from build123d import *

# Parameters (mm, degrees)
SKETCH1_R           = 5
BOSS_EXTRUDE1_DEPTH = 11
CUT_EXTRUDE1_DEPTH  = 8
BOSS_EXTRUDE2_DEPTH = 7


with BuildPart() as part:
    # Sketch1 → Boss-Extrude1 (new body)
    with BuildSketch(Plane.XY):
        with Locations((-12.317334514, -23.116112266)):
            Circle(SKETCH1_R)
    extrude(amount=BOSS_EXTRUDE1_DEPTH)

    # Sketch2 → Cut-Extrude1 (cut)
    with BuildSketch(Plane.XY.offset(11)):
        with BuildLine():
            Line((-14.317334514, -24.366112266), (-14.317334514, -21.866112266))
            ThreePointArc((-14.317334514, -21.866112266), (-12.317334514, -19.866112266), (-10.317334514, -21.866112266))
            Line((-10.317334514, -21.866112266), (-10.317334514, -24.366112266))
            ThreePointArc((-10.317334514, -24.366112266), (-12.317334514, -26.366112266), (-14.317334514, -24.366112266))
        make_face()
    extrude(amount=-CUT_EXTRUDE1_DEPTH, mode=Mode.SUBTRACT)

    # Sketch4 → Boss-Extrude2 (add)
    with BuildSketch(Plane(origin=(0, 0, 0), x_dir=(-1, 0, 0), z_dir=(0, 0, -1))):
        with BuildLine():
            Line((10.442334514, -24.116112266), (10.442334514, -22.116112266))
            ThreePointArc((10.442334514, -22.116112266), (12.317334514, -20.241112266), (14.192334514, -22.116112266))
            Line((14.192334514, -22.116112266), (14.192334514, -24.116112266))
            ThreePointArc((14.192334514, -24.116112266), (12.317334514, -25.991112266), (10.442334514, -24.116112266))
        make_face()
    extrude(amount=BOSS_EXTRUDE2_DEPTH)


solid = part.part
Here's how the part is built. I have some questions about the finished solid (model axes, mm). A direction names the side the tool comes from. Coordinates: 2 decimals unless noted, no trailing zeros. Write each loop counter-clockwise with the first axis right and the second up, starting at its lowest first coordinate (ties: lowest second). Pieces come first, ordered by that corner, then holes.
Item 1: I want a section at B-B on z = -4.75. Write out the boundary of the cut face in (x, y) (3 decimals), and give its area (3 significant figures).
Item 2: On a 3-axis mill with a long thin cutter (end or side, diameter ignored), from which of +Z, -Z, +X, -X, +Y, -Y can I reach the whole of each face in a straight line? I mean faces 1 (the flat face through (-12, -23, 3)), 2 (the flat face through (-14.192, -23, -3)), 3 (the cylindrical face through (-12.36, -25.99, -3.45)). Say none if no direction works.
Item 3: I want a section at A-A on x = -13.75. Write out the boundary of the cut face in (y, z).
Item 4: Will these pins go through, and if not, where does the flat tip stop? pin 1 (0.6 mm diameter, centred on y = -23.5, z = -2.5, fed in from +X); pin 2 (1.6 mm diameter, centred on y = -22.5, z = -4.5, fed in from -X); pin 3 (2 mm diameter, centred on x = -13, y = -23.5, fed in from +Z); pin 4 (1.2 mm diameter, centred on y = -22.5, z = 6.5, fed in from -X).
Item 5: If I drill on line 1 (Z direction, x = -11.75, y = -26.5); line 2 (Z direction, x = -13.25, y = -22.25); line 3 (Y direction, x = -13.25, z = 5.5), over which ranges is the centre line in solid material (lowest first)?
Item 6: I want a section at D-D on z = 9.5. Write out the boundary of the cut face in (x, y).
Item 7: I want a section at C-C on y = -25.5. Write out the boundary of the cut face in (x, z), and give its area (3 significant figures).
Item 8: If we mould it in two halves opening along Y, with no side actions, what happens to faces 4 (the cylindrical face through (-12.28, -20.24, -3.45)), 5 (the flat face through (-10.317, -23, 7)), 6 (the flat face through (-12, -23, -7))? For each: +Y half, -Y half, draft (parallel to the pull), parting line (faces both ways), or undercut.
Findings below:
1. outline: (-14.192, -24.116) arc R1.875 ccw to (-10.442, -24.116) - (-10.442, -22.116) arc R1.875 ccw to (-14.192, -22.116) - close
1. area: 18.5 mm2
2. face 1: +Z
2. face 2: -Z, -X, +Y, -Y
2. face 3: -Z, -Y
3. outline: (-27.91, 0) - (-25.33, 0) - (-25.33, -7) - (-20.91, -7) - (-20.91, 0) - (-18.33, 0) - (-18.33, 11) - (-20.47, 11) - (-20.47, 3) - (-25.76, 3) - (-25.76, 11) - (-27.91, 11) - close
4. pin 1: stops at x = -10.44
4. pin 2: stops at x = -14.19
4. pin 3: stops at z = 3
4. pin 4: stops at x = -17.32
5. line 1: z = 0 to 11
5. line 2: z = -7 to 3
5. line 3: y = -28.03 to -26.14, -20.1 to -18.2
6. outline: circle Ø10 at (-12.32, -23.12); hole (-14.32, -24.37) arc R2 ccw to (-10.32, -24.37) - (-10.32, -21.87) arc R2 ccw to (-14.32, -21.87) - close
7. outline: (-16.71, 0) - (-13.58, 0) - (-13.58, -7) - (-11.05, -7) - (-11.05, 0) - (-7.92, 0) - (-7.92, 11) - (-10.67, 11) - (-10.67, 3) - (-13.96, 3) - (-13.96, 11) - (-16.71, 11) - close
7. area: 88.0 mm2
8. face 4: +Y half
8. face 5: undercut
8. face 6: draft
